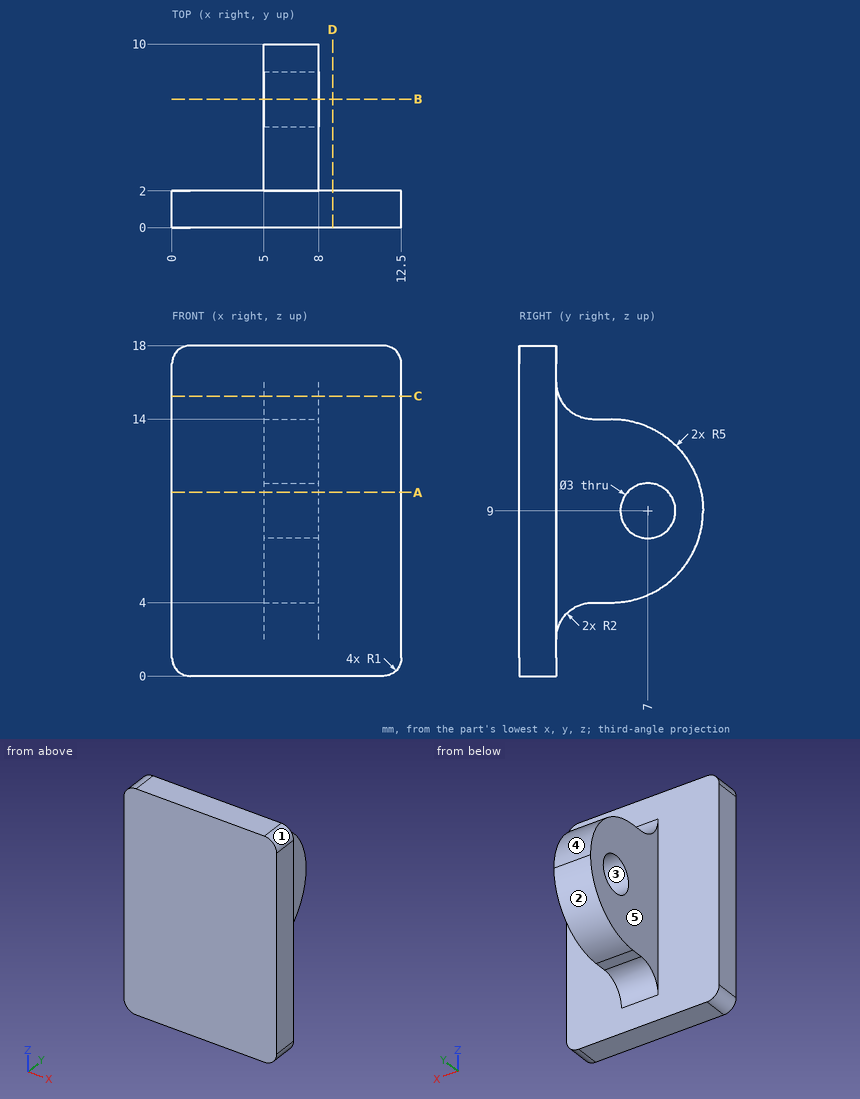
Job drawing, mm, ordinate dimensions from the low corner. One solid piece. A direction names the side the tool comes from. Round coordinates to 2 decimals unless told otherwise and drop trailing zeros. Write each loop counter-clockwise with the first axis right and the second up, starting at its lowest first coordinate (ties: lowest second). Pieces come first, ordered by that corner, then holes.
1) Band-saw the part on B-B, the plane y = 7. List the corners of the cut face in (x, z), and give its area (3 significant figures).
2) Band-saw the part on C-C, the plane z = 15.25. List the corners of the cut face in (x, y), and give its area (3 significant figures).
3) Band-saw the part on A-A, the plane z = 10. List the corners of the cut face in (x, y), and give its area (3 significant figures).
4) Mould opens along Z. For the marked faces 1, 2 and 3 say: +Z half, -Z half, draft (parallel to the pull), parting line (faces both ways), or undercut.
5) Drill centre lines: probe 1 along Y at (x, z) = (5.85, 9); probe 2 along Y at (x, z) = (10.5, 17.25); probe 3 along X at (y, z) = (4.25, 9.25). Where is each one in solid material? Low to high.
6) Band-saw the part on D-D, the plane x = 8.75. List the corners of the cut face in (y, z).
7) 3-axis set-ups, long thin cutter, end or side, ignore diameter. For the marked faces 4 and 5: which of +Z, -Z, +X, -X, +Y, -Y reach the whole face in a straight line?
8) Pin check, flat tips, straight feed: pin 1 (0.8 mm diameter, centred on x = 6, y = 4.5, fed in from -Z); pin 2 (2 mm diameter, centred on x = 6.5, y = 7, fed in from +Z); pin 3 (2.5 mm diameter, centred on y = 6, z = 11, fed in from -X). Stop position of each tip, or through.
Ans:
1. outline: (5, 4.42) - (8, 4.42) - (8, 7.5) - (5, 7.5) - close; (5, 10.5) - (8, 10.5) - (8, 13.58) - (5, 13.58) - close
1. area: 18.5 mm2
2. outline: (0, 0) - (12.5, 0) - (12.5, 2) - (8, 2) - (8, 2.15) - (5, 2.15) - (5, 2) - (0, 2) - close
2. area: 25.4 mm2
3. outline: (0, 0) - (12.5, 0) - (12.5, 2) - (8, 2) - (8, 5.88) - (5, 5.88) - (5, 2) - (0, 2) - close; (5, 8.12) - (8, 8.12) - (8, 9.9) - (5, 9.9) - close
3. area: 42.0 mm2
4. face 1: +Z half
4. face 2: -Z half
4. face 3: undercut
5. probe 1: y = 0 to 5.5, 8.5 to 10
5. probe 2: y = 0 to 2
5. probe 3: x = 5 to 8
6. outline: (0, 0) - (2, 0) - (2, 18) - (0, 18) - close
7. face 4: +Z, +X, -X, +Y
7. face 5: +Z, -Z, -X, +Y
8. pin 1: stops at z = 4
8. pin 2: stops at z = 13.9
8. pin 3: stops at x = 5
